Could you check a few things on this model? Use its own coordinates, in mm. A direction names the side the tool comes from. Coordinates: 2 decimals unless noted, no trailing zeros. Order: outer loops, then holes, each group sorted by start corner. A loop starts at its lowest first (then second) coordinate and runs counter-clockwise, first axis right, second up. Notation, with made-up numbers: (48.5, -30.5) - (68.5, -30.5) arc R20 cw to (68.5, 3.5) - close; hole circle Ø11 at (-17.5, 52.5). An arc over 180 degrees is marked (long way). One line per item, written item: value.
Autodesk Fusion 360 part; units mm, degrees
sketch "스케치1" plane through (0, 0, 0) normal (0, 0, 1) x (1, 0, 0)
  line L0 (0, 0) -> (44, 0)
  line L1 (0, 0) -> (0, 4)
  line L2 (0, 4) -> (41, 4)
  line L3 (0, 0) -> (44, 0)
  line L4 (44, 0) -> (100.5, 76)
  line L5 (100.5, 76) -> (97.5, 76)
  line L6 (44, 0) -> (41, 0)
  line L7 (41, 0) -> (97.5, 76)
  line L8 (41, 4) -> (43.9737, 4)
  line L9 (100.5, 76) -> (97.5, 76)
  line L10 (97.5, 76) -> (97.5, 176)
  line L11 (97.5, 176) -> (100.5, 176)
  line L12 (100.5, 176) -> (100.5, 76)
  line L13 (0, 4) -> (0, 76)
  line L14 (0, 76) -> (7.5, 76)
  line L15 (7.5, 76) -> (12.5, 76)
  line L16 (12.5, 76) -> (12.5, 96)
  line L17 (12.5, 96) -> (7.5, 96)
  line L18 (7.5, 96) -> (7.5, 76)
  line L19 (97.5, 176) -> (12.5, 176)
  line L20 (12.5, 176) -> (12.5, 173)
  line L21 (12.5, 173) -> (97.5, 173)
  line L22 (97.5, 173) -> (97.5, 176)
  line L23 (12.5, 176) -> (7.5, 176)
  line L24 (7.5, 176) -> (7.5, 153)
  line L25 (7.5, 153) -> (12.5, 153)
  line L26 (12.5, 153) -> (12.5, 176)
  dimension "d1" = 44
  dimension "d2" = 4
  dimension "d3" = 41
  dimension "d7" = 3
  dimension "d8" = 3
  dimension "d9" = 3
  dimension "d10" = 100
  dimension "d19" = 72
  dimension "d20" = 7.5
  dimension "d21" = 5
  dimension "d22" = 20
  dimension "d26" = 85
  dimension "d27" = 3
  dimension "d28" = 23
extrude "돌출1" add sketch "스케치1" along normal blind 105 makes body 1 at (100.5, 142.6667, 35) makes body 2 at (7.5, 89.3333, 35)
sketch "스케치2" plane through (0, 0, 105) normal (0, 0, 1) x (-1, 0, 0)
  line L0 (0, 0) -> (-44, 0)
  line L1 (-44, 0) -> (-100.5, -76)
  line L2 (-100.5, -76) -> (-100.5, -176)
  line L3 (-100.5, -176) -> (-7.5, -176)
  line L4 (-97.5, -173) -> (-97.5, -76)
  line L5 (-97.5, -76) -> (-43.9737, -4)
  line L6 (-43.9737, -4) -> (0, -4)
  line L7 (0, -4) -> (0, 0)
  line L8 (0, -4) -> (0, -176)
  line L9 (0, -176) -> (-7.5, -176)
  line L10 (-12.5, -153) -> (-12.5, -173)
  line L11 (-12.5, -173) -> (-97.5, -173)
  line L12 (-7.5, -176) -> (-7.5, -153)
  line L13 (-7.5, -153) -> (-12.5, -153)
extrude "돌출2" add sketch "스케치2" against normal blind 3 contours L4 L5 L6 L8 L9 L10 L11 L12 L13 bodies 1 2
fillet "필렛1" radius 10 2 edges at (100.5, 76, 52.5) (44, 0, 52.5) on bodies 1
fillet "필렛2" radius 2.5 5 edges at (19.4868, 0, 105) (43.4646, 1.0652, 105) (72.7621, 38.6888, 105) (99.9935, 76.1676, 105) (100.5, 127.6549, 105) on bodies 1
sketch "스케치3" plane through (0, 173, 0) normal (0, -1, 0) x (1, 0, 0)
  line L0 (97.5, 102) -> (12.5, 102)
  line L1 (12.5, 102) -> (12.5, 0)
  line L2 (12.5, 0) -> (97.5, 0)
  line L3 (97.5, 0) -> (97.5, 102)
  line L4 (97.5, 0) -> (94.5, 0)
  line L5 (94.5, 0) -> (94.5, 3)
  line L6 (94.5, 3) -> (97.5, 3)
  line L7 (97.5, 3) -> (97.5, 0)
  line L8 (12.5, 102) -> (15.5, 102)
  line L9 (15.5, 102) -> (15.5, 99)
  line L10 (15.5, 99) -> (12.5, 99)
  line L11 (12.5, 99) -> (12.5, 102)
  line L12 (15.5, 99) -> (94.5, 99)
  line L13 (94.5, 99) -> (94.5, 3)
  line L14 (94.5, 3) -> (15.5, 3)
  line L15 (15.5, 3) -> (15.5, 99)
  line L16 (94.5, 99) -> (94.5, 56)
  line L17 (94.5, 56) -> (84.5, 56)
  line L18 (84.5, 56) -> (84.5, 46)
  line L19 (84.5, 46) -> (94.5, 46)
  line L20 (94.5, 46) -> (94.5, 56)
  line L21 (15.5, 56) -> (25.5, 56)
  line L22 (25.5, 56) -> (25.5, 46)
  line L23 (25.5, 46) -> (15.5, 46)
  line L24 (15.5, 46) -> (15.5, 56)
  circle A0 centre (89.5, 51) radius 2.15
  circle A1 centre (20.5, 51) radius 2.15
  dimension "d29" = 3
  dimension "d30" = 3
  dimension "d31" = 3
  dimension "d32" = 3
  dimension "d35" = 43
  dimension "d36" = 10
  dimension "d37" = 10
  dimension "d38" = 10
  dimension "d39" = 10
  dimension "d40" = 4.3
  dimension "d41" = 4.3
extrude "돌출3" cut sketch "스케치3" against normal blind 3 contours L12 L13 L14 L15 L16 L17 L18 L19 L21 L22 L23 | A0 | A1 bodies 1
sketch "스케치4" plane through (7.5, 0, 0) normal (-1, 0, 0) x (0, -1, 0)
  line L0 (-153, 102) -> (-176, 102)
  line L1 (-176, 102) -> (-176, 0)
  line L2 (-176, 0) -> (-153, 0)
  line L3 (-153, 0) -> (-153, 102)
  line L4 (-153, 102) -> (-153, 73)
  line L5 (-153, 73) -> (-173, 73)
  line L6 (-173, 73) -> (-173, 53)
  line L7 (-173, 53) -> (-153, 53)
  line L8 (-153, 53) -> (-153, 73)
  circle A0 centre (-163, 63) radius 2.65
  dimension "d42" = 29
  dimension "d43" = 20
  dimension "d44" = 20
  dimension "d45" = 5.3
sketch "스케치5" plane through (7.5, 0, 0) normal (-1, 0, 0) x (0, -1, 0)
  line L0 (-76, 102) -> (-96, 102)
  line L1 (-96, 102) -> (-96, 0)
  line L2 (-96, 0) -> (-76, 0)
  line L3 (-76, 0) -> (-76, 102)
  line L4 (-76, 102) -> (-76, 53)
  line L5 (-76, 53) -> (-96, 53)
  line L6 (-96, 53) -> (-96, 33)
  line L7 (-96, 33) -> (-76, 33)
  line L8 (-76, 33) -> (-76, 53)
  circle A0 centre (-86, 43) radius 2.65
  dimension "d46" = 49
  dimension "d47" = 20
  dimension "d48" = 5.3
extrude "돌출4" cut sketch "스케치4" sketch "스케치5" against normal blind 5 contours A0 of sketch 2 contours A0 bodies 1
sketch "스케치6" plane through (0, 0, 102) normal (0, 0, -1) x (1, 0, 0)
  line L0 (7.5, -176) -> (7.5, -153)
  line L1 (7.5, -153) -> (12.5, -153)
  line L2 (12.5, -153) -> (12.5, -173)
  line L3 (12.5, -173) -> (97.5, -173)
  line L4 (97.5, -173) -> (97.5, -76)
  line L5 (97.5, -76) -> (43.9737, -4)
  line L6 (43.9737, -4) -> (0, -4)
  line L7 (0, -4) -> (0, -176)
  line L8 (0, -176) -> (7.5, -176)
  line L9 (12.5, -96) -> (7.5, -96)
  line L10 (7.5, -96) -> (7.5, -76)
  line L11 (7.5, -76) -> (12.5, -76)
  line L12 (12.5, -76) -> (12.5, -96)
  line L13 (0, -76) -> (7.5, -76)
  line L14 (7.5, -76) -> (7.5, -176)
  line L15 (7.5, -176) -> (0, -176)
  line L16 (0, -176) -> (0, -76)
extrude "돌출5" cut sketch "스케치6" against normal blind 3 contours L0 L7 L8 L10 L13 L14 L15 L16 bodies 1
sketch "스케치7" plane through (0, 4, 0) normal (0, 1, 0) x (-1, 0, 0)
  line L0 (0, 102) -> (-43.9737, 102)
  line L1 (-43.9737, 102) -> (-43.9737, 0)
  line L2 (-43.9737, 0) -> (0, 0)
  line L3 (0, 0) -> (0, 102)
  line L4 (0, 0) -> (0, 28)
  line L5 (0, 28) -> (-3, 28)
  line L6 (-3, 28) -> (-3, 38)
  line L7 (-3, 38) -> (0, 38)
  line L8 (0, 38) -> (0, 28)
  dimension "d53" = 28
  dimension "d54" = 3
  dimension "d55" = 10
extrude "돌출6" add sketch "스케치7" along normal blind 13 contours L3 L5 L6 L7 L8 bodies 1
sketch "스케치8" plane through (0, 0, 0) normal (-1, 0, 0) x (0, -1, 0)
  line L0 (-76, 105) -> (-76, 102)
  line L1 (-76, 102) -> (-4, 102)
  line L2 (-4, 102) -> (-4, 38)
  line L3 (-4, 38) -> (-17, 38)
  line L4 (-17, 38) -> (-17, 28)
  line L5 (-17, 28) -> (-4, 28)
  line L6 (-4, 28) -> (-4, 0)
  line L7 (-4, 0) -> (0, 0)
  line L8 (0, 0) -> (0, 102.5)
  arc A0 (0, 102.5) -> (-2.5, 105) centre (-2.5, 102.5) ccw
  line L9 (-2.5, 105) -> (-76, 105)
  line L10 (-17, 38) -> (-7, 38)
  line L11 (-7, 38) -> (-7, 28)
  line L12 (-7, 28) -> (-17, 28)
  line L13 (-17, 28) -> (-17, 38)
  circle A1 centre (-12, 33) radius 2.15
  dimension "d58" = 4.3
extrude "돌출7" cut sketch "스케치8" against normal blind 3 contours A1 bodies 1
sketch "스케치9" plane through (0, 0, 102) normal (0, 0, -1) x (1, 0, 0)
  line L0 (7.5, -96) -> (7.5, -153)
  line L1 (7.5, -153) -> (12.5, -153)
  line L2 (12.5, -153) -> (12.5, -173)
  line L3 (12.5, -173) -> (97.5, -173)
  line L4 (97.5, -173) -> (97.5, -76)
  line L5 (97.5, -76) -> (43.9737, -4)
  line L6 (43.9737, -4) -> (0, -4)
  line L7 (0, -4) -> (0, -76)
  line L8 (0, -76) -> (7.5, -76)
  line L9 (7.5, -76) -> (12.5, -76)
  line L10 (12.5, -76) -> (12.5, -96)
  line L11 (12.5, -96) -> (7.5, -96)
  line L12 (0, -4) -> (3, -4)
  line L13 (3, -4) -> (3, -10)
  line L14 (3, -10) -> (0, -10)
  line L15 (0, -10) -> (0, -4)
  dimension "d61" = 3
  dimension "d62" = 6
extrude "돌출8" add sketch "스케치9" along normal blind 64 contours L6 L7 L12 L13 L14 L15 bodies 1
sketch "스케치10" plane through (0, 0, 28) normal (0, 0, -1) x (1, 0, 0)
  line L0 (3, -4) -> (0, -4)
  line L1 (0, -4) -> (0, -17)
  line L2 (0, -17) -> (3, -17)
  line L3 (3, -17) -> (3, -4)
  line L4 (0, -4) -> (3, -4)
  line L5 (3, -4) -> (3, -10)
  line L6 (3, -10) -> (0, -10)
  line L7 (0, -10) -> (0, -4)
  dimension "d65" = 6
extrude "돌출9" add sketch "스케치10" along normal blind 28 contours L0 L1 L3 L4 L5 L6 L7 bodies 1
mirror "미러1" about plane through (0, 0, 0) normal (1, 0, 0) of bodies 1 makes body 3
hidden bodies 1
Item 1: If I drill on probe 1 along Z at (x, y) = (-89.5, 173.9); probe 2 along Y at (x, z) = (-11, 36); probe 3 along X at (y, z) = (106, 45), over which ranges is the centre line in solid material (lowest first)?
Conclusion:
probe 1: 0 to 3, 46 to 48.85, 53.15 to 56, 99 to 105
probe 2: 0 to 4, 76 to 96, 153 to 176
probe 3: -100.5 to -97.5
Item 2: I want a section at A-A on y = 86. Please give me the cut outline in (x, z).
Conclusion:
outline: (-100.5, 0) - (-97.5, 0) - (-97.5, 102) - (-12.5, 102) - (-12.5, 45.65) - (-7.5, 45.65) - (-7.5, 105) - (-98, 105) arc R2.5 ccw to (-100.5, 102.5) - close; (-12.5, 0) - (-7.5, 0) - (-7.5, 40.35) - (-12.5, 40.35) - close
Item 3: I want a section at C-C on z = 51. Give the number of separate pieces and of enclosed holes in the cut face, then the cut area to 3 significant figures.
Conclusion:
separate pieces: 5
enclosed holes: 0
area: 978 mm²
Item 4: I'm going to push flat-ended pins straight in: pin 1 Ø1.5 at (x, z) = (-1.5, 8.5) entering from +Y; pin 2 Ø1.5 at (x, z) = (-2, 35) entering from +Y; pin 3 Ø0.9 at (x, z) = (-3.5, 103.5) entering from +Y. Where does each tip first touch, or does it pass through?
Conclusion:
pin 1: y = 10
pin 2: y = 17
pin 3: y = 76
Item 5: For faces 5 (the face through (-10, 76, 50)), 6 (the face through (-3, 8, 52)), 7 (the face through (-7.5, 159, 52)), 8 (the face through (-97.5, 125, 50)), which set-ups out of +Z, -Z, +X, -X, +Y, -Y let a thin tool reach every point of the face, with its end or its side?
Conclusion:
face 5: -Z, +X
face 6: -Z, +Y
face 7: +Z, -Z, +X, +Y
face 8: -Z
Item 6: I want a section at D-D on x = -20.5. Please give me the cut outline in (y, z).
Conclusion:
outline: (0, 0) - (4, 0) - (4, 102) - (173, 102) - (173, 99) - (176, 99) - (176, 105) - (2.5, 105) arc R2.5 ccw to (0, 102.5) - close; (173, 0) - (176, 0) - (176, 3) - (173, 3) - close; (173, 46) - (176, 46) - (176, 48.85) - (173, 48.85) - close; (173, 53.15) - (176, 53.15) - (176, 56) - (173, 56) - close
Item 7: Thinking about a two-plate mould opening in Z: for faces 1 (the face through (-10, 153, 50)), 2 (the face through (-21.66, 174.48, 49.19)), 3 (the face through (-71.798, 38.652, 104.287)), 4 (the face through (-10, 86, 0)), which applies, pulls with the +Z half, pulls with the -Z half, needs draft (parallel to the pull), parting line crosses it, or undercut?
Conclusion:
face 1: needs draft
face 2: undercut
face 3: pulls with the +Z half
face 4: pulls with the -Z half
Item 8: I want a section at B-B on z = 87. Please give me the cut outline in (x, y), then the cut area to 3 significant figures.
Conclusion:
outline: (-100.5, 79.31) arc R10 ccw to (-98.53, 73.34) - (-47, 4.03) arc R10 ccw to (-38.97, 0) - (0, 0) - (0, 10) - (-3, 10) - (-3, 4) - (-43.97, 4) - (-97.5, 76) - (-97.5, 173) - (-94.5, 173) - (-94.5, 176) - (-100.5, 176) - close; (-15.5, 173) - (-12.5, 173) - (-12.5, 153) - (-7.5, 153) - (-7.5, 176) - (-15.5, 176) - close; (-12.5, 76) - (-7.5, 76) - (-7.5, 96) - (-12.5, 96) - close
area: 944 mm²
